from build123d import *

# Parameters (mm, degrees)
SKIZZE1_R                       = 14
AUFSATZ_LINEAR_AUSTRAGEN1_DEPTH = 40
SKIZZE2_R                       = 5
AUFSATZ_LINEAR_AUSTRAGEN2_DEPTH = 16
SKIZZE3_R                       = 5
AUFSATZ_LINEAR_AUSTRAGEN3_DEPTH = 10
AUFSATZ_LINEAR_AUSTRAGEN3_TAPER = 10


with BuildPart() as part:
    # Skizze1 → Aufsatz-Linear austragen1 (new body)
    with BuildSketch(Plane.XY):
        Circle(SKIZZE1_R)
    extrude(amount=AUFSATZ_LINEAR_AUSTRAGEN1_DEPTH)

    # Skizze2 → Aufsatz-Linear austragen2 (add)
    with BuildSketch(Plane(origin=(0, 0, 0), x_dir=(-1, 0, 0), z_dir=(0, 0, -1))):
        Circle(SKIZZE2_R)
    extrude(amount=AUFSATZ_LINEAR_AUSTRAGEN2_DEPTH)

    # Skizze3 → Aufsatz-Linear austragen3 (add)
    with BuildSketch(Plane.XY.offset(40)):
        with Locations((0, -0.81713022)):
            Circle(SKIZZE3_R)
    extrude(amount=AUFSATZ_LINEAR_AUSTRAGEN3_DEPTH, taper=AUFSATZ_LINEAR_AUSTRAGEN3_TAPER)


solid = part.part
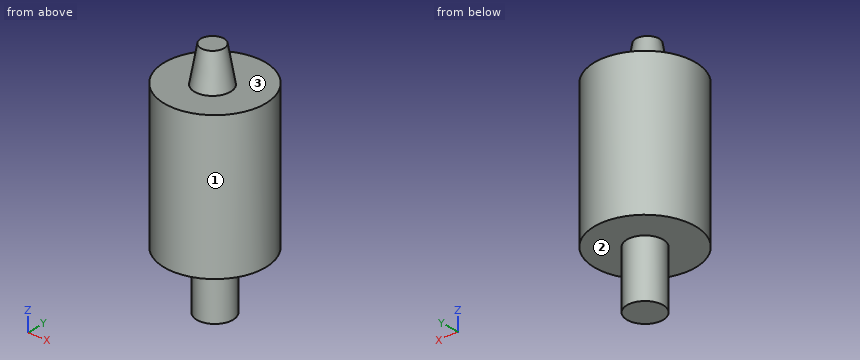
Can you work these out from the model? Positions are in its coordinate system, mm. Face numbers are marked on the shaded views. A direction names the side the tool comes from. Give positions to 0.01 mm unless a question says otherwise; leave off trailing zeros. Write each loop counter-clockwise with the first axis right and the second up, starting at its lowest first coordinate (ties: lowest second). Pieces come first, ordered by that corner, then holes. Notation, with made-up numbers: M 67,-11 L 90,-11 A12 cw 90,12 Z; hole C 20.25,41 d4. An arc over 180 degrees is marked long. Answer in a Markdown table with one row per item. Add a question column.
Item 1: Imagine slicing it at D-D, the plane z = 21.5. Write out the boundary of the cut face in (x, y).
Item 2: For pin 1 Ø5 at (y, z) = (5.5, -1) entering from -X; pin 2 Ø2 at (y, z) = (-7.5, 17.5) entering from +X; pin 3 Ø3 at (y, z) = (2, 35) entering from +X, each with a flat end and sliding along its axis, tell me the tip position at first contact or that it passes through.
Item 3: Imagine slicing it at A-A, the plane x = 0. Write out the boundary of the cut face in (y, z), plus the area to 3 significant figures.
Item 4: On a 3-axis mill with a long thin cutter (end or side, diameter ignored), from which of +Z, -Z, +X, -X, +Y, -Y can I reach the whole of each face in a straight line? I mean the marked faces 1, 2 and 3. Say none if no direction works.
Item 5: Please list where these lines run through material, in increasing order: L1, parallel to Z at x = 3, y = 3.5; L2, parallel to Z at x = 10.5, y = -6.75; L3, parallel to Y at x = 10.5, z = 1.5.
Item 6: Imagine slicing it at B-B, the plane z = -9. Write out the boundary of the cut face in (x, y), plus the area to 3 significant figures.
Item 7: Imagine slicing it at C-C, the plane y = 10.25. Write out the boundary of the cut face in (x, z), plus the area to 3 significant figures.
Evaluation:
| question | item | result |
|---|---|---|
| 1 | outline | C 0,0 d28 |
| 2 | pin 1 | stops at x = -13.63 |
| 2 | pin 2 | stops at x = 12.4 |
| 2 | pin 3 | stops at x = 13.99 |
| 3 | outline | M -14,0 L -5,0 L -5,-16 L 5,-16 L 5,0 L 14,0 L 14,40 L 4.18,40 L 2.42,50 L -4.05,50 L -5.82,40 L -14,40 Z |
| 3 | area | 1,360 mm² |
| 4 | face 1 | +Z, -Z |
| 4 | face 2 | -Z |
| 4 | face 3 | +Z |
| 5 | L1 | z = -16 to 40 |
| 5 | L2 | z = 0 to 40 |
| 5 | L3 | y = -9.26 to 9.26 |
| 6 | outline | C 0,0 d10 |
| 6 | area | 78.5 mm² |
| 7 | outline | M -9.54,0 L 9.54,0 L 9.54,40 L -9.54,40 Z |
| 7 | area | 763 mm² |
